Autodesk Inventor part; units mm, degrees
ref_plane "YZ Plane" through (0, 0, 0) normal (1, 0, 0) x (0, 1, 0)
ref_plane "XZ Plane" through (0, 0, 0) normal (0, 1, 0) x (-1, 0, 0)
ref_plane "XY Plane" through (0, 0, 0) normal (0, 0, 1) x (1, 0, 0)
sketch "Sketch1" plane through (0, 0, 0) normal (0, 1, 0) x (-1, 0, 0)
  line L0 (-30, 11) -> (-6, 11)
  line L1 (30, 11) -> (30, 2.5)
  line L2 (30, -11) -> (-30, -11)
  line L3 (-30, -11) -> (-30, 11)
  line L4 (-30, 11) -> (30, -11) construction
  line L5 (30, 11) -> (-30, -11) construction
  line L6 (6, 11) -> (6, 1)
  line L7 (-6, 1) -> (-6, 11)
  arc A0 (-6, 1) -> (6, 1) centre (0, 1) ccw
  line L8 (-20, 1) -> (-25, 1) construction
  line L9 (-20, 2.5) -> (-25, 2.5)
  line L10 (-25, -0.5) -> (-20, -0.5)
  arc A1 (-20, -0.5) -> (-20, 2.5) centre (-20, 1) ccw
  arc A2 (-25, 2.5) -> (-25, -0.5) centre (-25, 1) ccw
  line L11 (30, 1) -> (25, 1) construction
  line L12 (30, 2.5) -> (25, 2.5)
  line L13 (25, -0.5) -> (30, -0.5)
  arc A3 (30, -0.5) -> (30, 2.5) centre (30, 1) ccw construction
  arc A4 (25, 2.5) -> (25, -0.5) centre (25, 1) ccw
  line L14 (30, -0.5) -> (30, -11)
  line L15 (30, 2.5) -> (30, -0.5) construction
  line L16 (6, 11) -> (30, 11)
  line L17 (-6, 11) -> (6, 11) construction
  point P0 (0, 0)
  point P1 (0, 0)
  point P2 (0, 0)
  point P3 (-22.5, 1)
  point P4 (27.5, 1)
  dimension "d0" = 60
  dimension "d1" = 22
  dimension "d3" = 1
  dimension "d4" = 12
  dimension "d5" = 5
  dimension "d6" = 3
  dimension "d7" = 10
  dimension "d8" = 5
  dimension "d9" = 5
extrude "Extrusion1" add sketch "Sketch1" along normal mid plane 2.5
fillet "Fillet1" radius 2 4 edges at (-30, 0, -11) (-30, 0, 11) (30, 0, -11) (30, 0, 11)
fillet "Fillet1" radius 1 2 edges at (-6, 0, 11) (6, 0, 11)
fillet "Fillet2" radius 0.25 30 edges at (0, 1.25, -5) (6, 1.25, 5.5) (6.2929, 1.25, 10.7071) (17.5, 1.25, 11) (29.4142, 1.25, 10.4142) (30, 1.25, 0) (29.4142, 1.25, -10.4142) (0, 1.25, -11) (-29.4142, 1.25, -10.4142) (-30, 1.25, -4.75) (-6.2929, 1.25, 10.7071) (-17.5, 1.25, 11) (-29.4142, 1.25, 10.4142) (-30, 1.25, 5.75) (-6, 1.25, 5.5) (-6.2929, -1.25, 10.7071) (-17.5, -1.25, 11) (-29.4142, -1.25, 10.4142) (-30, -1.25, 5.75) (0, -1.25, -5) (6, -1.25, 5.5) (6.2929, -1.25, 10.7071) (17.5, -1.25, 11) (29.4142, -1.25, 10.4142) (30, -1.25, 0) (29.4142, -1.25, -10.4142) (0, -1.25, -11) (-29.4142, -1.25, -10.4142) (-30, -1.25, -4.75) (-6, -1.25, 5.5)
equation "\"d8\" = d5"
properties part number "Extruder Plate" material "Stainless Steel"
Geometry check sheet. Reference: the model listing, model coordinates, mm. A direction names the side the tool comes from. Give positions to 0.01 mm unless a question says otherwise; leave off trailing zeros. Write each loop counter-clockwise with the first axis right and the second up, starting at its lowest first coordinate (ties: lowest second). Pieces come first, ordered by that corner, then holes.
1) Section check B-B, the plane y = -0.15. Record the boundary of the cut face in (x, z).
2) Section check C-C, the plane x = 0. Record the boundary of the cut face in (y, z), and give its area (3 significant figures).
3) Access from +Z, -Z, +X, -X, +Y, -Y to the whole of each face (thin tool, end or side, straight path). Record for faces 4 (the flat face through (6, 0, 5)), 5 (the flat face through (22, 0, 2.5)), 6 (the flat face through (0, 0, -11)), 7 (the flat face through (-17, 0, 11)), 8 (the flat face through (-28, 0, 2.5)).
4) Material ranges on L1, parallel to X at y = -0.25, z = 0; L2, parallel to X at y = -0.95, z = 5.75; L3, parallel to Z at x = 22.5, y = -0.1, recorded low to high.
5) Release check for a two-part mould opening along X. For faces 1 (the cylindrical face through (-6.285, -0.014, 10.699)), 2 (the cylindrical face through (29.43, 0.01, -10.4)), 3 (the flat face through (7, 1.25, 0)) record: pulls with the +X half, pulls with the -X half, needs draft (parallel to the pull), parting line crosses it, or undercut.
6) Section check A-A, the plane x = 21.5. Record the boundary of the cut face in (y, z), and give its area (3 significant figures).
Computed:
1. outline: (-30, -9) arc R2 ccw to (-28, -11) - (28, -11) arc R2 ccw to (30, -9) - (30, 9) arc R2 ccw to (28, 11) - (7, 11) arc R1 ccw to (6, 10) - (6, 1) arc R6 cw to (-6, 1) - (-6, 10) arc R1 ccw to (-7, 11) - (-28, 11) arc R2 ccw to (-30, 9) - (-30, 2.5) - (-25, 2.5) arc R1.5 cw to (-25, -0.5) - (-30, -0.5) - close; hole (20, -0.5) - (25, -0.5) arc R1.5 ccw to (25, 2.5) - (20, 2.5) arc R1.5 ccw to start
2. outline: (-1.25, -10.75) arc R0.25 ccw to (-1, -11) - (1, -11) arc R0.25 ccw to (1.25, -10.75) - (1.25, -5.25) arc R0.25 ccw to (1, -5) - (-1, -5) arc R0.25 ccw to (-1.25, -5.25) - close
2. area: 14.9 mm2
3. face 4: +Z, +Y, -Y
3. face 5: +Y, -Y
3. face 6: -Z, +X, -X, +Y, -Y
3. face 7: +Z, +X, -X, +Y, -Y
3. face 8: -X, +Y, -Y
4. L1: x = -23.88 to -5.92, 5.92 to 18.88, 26.12 to 30
4. L2: x = -30 to -6, 6 to 30
4. L3: z = -11 to -0.5, 2.5 to 11
5. face 1: undercut
5. face 2: pulls with the +X half
5. face 3: needs draft
6. outline: (-1.25, -10.75) arc R0.25 ccw to (-1, -11) - (1, -11) arc R0.25 ccw to (1.25, -10.75) - (1.25, -0.5) - (-1.25, -0.5) - close; (-1.25, 2.5) - (1.25, 2.5) - (1.25, 10.75) arc R0.25 ccw to (1, 11) - (-1, 11) arc R0.25 ccw to (-1.25, 10.75) - close
6. area: 47.4 mm2
